CAD build for the part. Positions are in the model's coordinates, mm. Coordinates: 2 decimals unless noted, no trailing zeros. Order: outer loops, then holes, each group sorted by start corner. A loop starts at its lowest first (then second) coordinate and runs counter-clockwise, first axis right, second up. Notation, with made-up numbers: M 66,-12.5 L 77,-12.5 A17 cw 77,19.5 Z; hole C 66,-3 d6. An arc over 180 degrees is marked long. Write item = value, one per line.
from build123d import *

# Parameters (mm, degrees)
ESQUISSE1_W             = 390
ESQUISSE1_H             = 355
BOSS_EXTRU_1_DEPTH      = 5
ESQUISSE3_W             = 80.434472185
ESQUISSE3_H             = 102.5
ESQUISSE3_H_2           = 103.87880101
ESQUISSE3_W_2           = 25.03
ESQUISSE3_H_3           = 25.03
ENL_V_MAT_EXTRU_1_DEPTH = 10
ESQUISSE4_W             = 80.434472185
ESQUISSE4_H             = 5
BOSS_EXTRU_2_DEPTH      = 1.38
ESQUISSE9_R             = 1.5
ENL_V_MAT_EXTRU_2_DEPTH = 264.735189158


with BuildPart() as part:
    # Esquisse1 → Boss.-Extru.1 (new body)
    with BuildSketch(Plane.XY):
        Rectangle(ESQUISSE1_W, ESQUISSE1_H)
    extrude(amount=BOSS_EXTRU_1_DEPTH)

    # Esquisse3 → Enlèv. mat.-Extru.1 (cut)
    with BuildSketch(Plane(origin=(0, 0, 0), x_dir=(-1, 0, 0), z_dir=(0, 0, -1))):
        with Locations((154.782763907, 78.25)):
            Rectangle(ESQUISSE3_W, ESQUISSE3_H)
        with Locations((154.782763907, -36.560599495)):
            Rectangle(ESQUISSE3_W, ESQUISSE3_H_2)
        with Locations((-182.485, 164.985)):
            Rectangle(ESQUISSE3_W_2, ESQUISSE3_H_3)
        with Locations((182.485, 164.985)):
            Rectangle(ESQUISSE3_W_2, ESQUISSE3_H_3)
        with Locations((182.485, -164.985)):
            Rectangle(ESQUISSE3_W_2, ESQUISSE3_H_3)
        with Locations((-182.485, -164.985)):
            Rectangle(ESQUISSE3_W_2, ESQUISSE3_H_3)
    extrude(amount=-ENL_V_MAT_EXTRU_1_DEPTH, mode=Mode.SUBTRACT)

    # Esquisse4 → Boss.-Extru.2 (add)
    with BuildSketch(Plane.XZ.offset(-15.37880101)):
        with Locations((-154.782763907, 2.5)):
            Rectangle(ESQUISSE4_W, ESQUISSE4_H)
    extrude(amount=BOSS_EXTRU_2_DEPTH)

    # Esquisse9 → Enlèv. mat.-Extru.2 (cut, through all)
    with BuildSketch(Plane(origin=(0, 0, 0), x_dir=(-1, 0, 0), z_dir=(0, 0, -1))):
        with Locations((175, -99.5)):
            Circle(ESQUISSE9_R)
        with Locations(Location((95, -99.5, 0), (0, 0, 180))):
            Circle(ESQUISSE9_R)
        with Locations((95, 140.5)):
            Circle(ESQUISSE9_R)
        with Locations(Location((175, 140.5, 0), (0, 0, 180))):
            Circle(ESQUISSE9_R)
    extrude(amount=-ENL_V_MAT_EXTRU_2_DEPTH, mode=Mode.SUBTRACT)


solid = part.part
(1) Wall check: line 1 (X direction, y = 140.5, z = 2.95); line 2 (Y direction, x = -126, z = 3.6); line 3 (Y direction, x = -175, z = 2.7). Give the ranges that are in metal, low to high. Write a range as from..to.
Evaluation:
line_1 = -195..-176.5, -173.5..-96.5, -93.5..195
line_2 = -177.5..-88.5, 14..27, 129.5..177.5
line_3 = -152.47..-101, -98..-88.5, 14..27, 129.5..139, 142..152.47
(2) Slice it at B-B, the plane y = 124.5. Write the cut outline in (x, z).
Evaluation:
outline = M -114.57,0 L 195,0 L 195,5 L -114.57,5 Z
(3) Pin check, flat tips, straight feed: pin 1 Ø1.5 at (x, z) = (187, 3.5) entering from +Y; pin 2 Ø10 at (x, y) = (-84, -134) entering from -Z; pin 3 Ø2.5 at (y, z) = (159.5, 3) entering from -X. Stop position of each tip, or through.
Evaluation:
pin_1 = 152.47
pin_2 = 0
pin_3 = -169.97
(4) Slice it at A-A, the plane z = 3.3. Write the cut outline in (x, y), then the cut area to 3 significant figures.
Evaluation:
outline = M -195,-152.47 L -169.97,-152.47 L -169.97,-177.5 L 169.97,-177.5 L 169.97,-152.47 L 195,-152.47 L 195,152.47 L 169.97,152.47 L 169.97,177.5 L -169.97,177.5 L -169.97,152.47 L -195,152.47 L -195,129.5 L -114.57,129.5 L -114.57,27 L -195,27 L -195,14 L -114.57,14 L -114.57,-88.5 L -195,-88.5 Z; hole C -175,-99.5 d3; hole C -175,140.5 d3; hole C -95,-99.5 d3; hole C -95,140.5 d3
area = 119,000 mm²
